The listing builds one solid part. Answer for the finished solid, in the listing's coordinates (mm). Face numbers are marked on the shaded views. A direction names the side the tool comes from. Coordinates: 2 decimals unless noted, no trailing zeros. Order: outer loops, then holes, each group sorted by start corner. A loop starts at its lowest first (then second) coordinate and runs counter-clockwise, first axis right, second up. Notation, with made-up numbers: (-40, 80) -> (10, 80) arc R19 ccw to (10, 105) -> close; hole circle Ø3 at (37.5, 49.5). An arc over 180 degrees is marked (long way). Answer in a Markdown table with one row per item.
```python
from build123d import *

# Parameters (mm, degrees)
F1_DEPTH = 32
F2_R     = 43.740238
F2_R_2   = 35
F3_DEPTH = 88.001
F4_SIZE2 = 10
F4_SIZE  = 10


with BuildPart() as f1:
    # F0 (on Front) → F1 (new body)
    with BuildSketch(Plane.XZ):
        Polygon((-12.5, 32), (-31.5, 32), (-31.5, -19), (-56.5, -19), (-56.5, -32), (-17.5, -32), (-17.5, -15), (17.5, -15), (17.5, -32), (56.5, -32), (56.5, -19), (31.5, -19), (31.5, 32), (12.5, 32), (12.5, -2), (-12.5, -2), align=None)
    extrude(amount=F1_DEPTH)

    # F2 (on face) → F3 (cut, through all)
    with BuildSketch(Plane.YZ.offset(31.5)):
        with Locations((-16, -3)):
            Circle(F2_R)
        with Locations((-16, -3)):
            Circle(F2_R_2, mode=Mode.SUBTRACT)
    extrude(amount=-F3_DEPTH, mode=Mode.SUBTRACT)

    # F4
    f4_edges = [f1.edges().sort_by_distance(p)[0] for p in [
        (-56.5, -32, -25.5),
        (56.5, -32, -25.5),
    ]]
    chamfer(f4_edges, length=F4_SIZE, length2=F4_SIZE2)


solid = f1.part
```
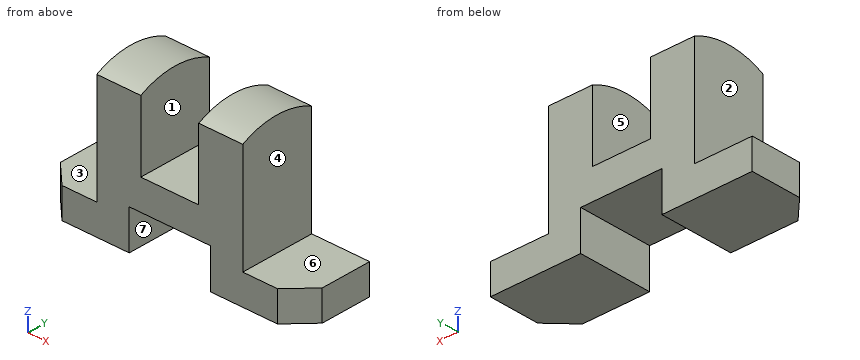
(1) Find the intervals of material crossed by line 1 along X through (y, z) = (-14.5, -18.5); line 2 along X through (y, z) = (-7, 20); line 3 along Z through (x, y) = (34, -25), in increasing order. Write a range as from..to.
Check values:
| item | result |
|---|---|
| line 1 | -31.5..-17.5, 17.5..31.5 |
| line 2 | -31.5..-12.5, 12.5..31.5 |
| line 3 | -32..-19 |
(2) A cutting plane is placed at C-C, the plane z = 15. Determine the outline of the cut face in (x, y), then the cut area to 3 significant figures.
Check values:
| item | result |
|---|---|
| outline | (-31.5, -32) -> (-12.5, -32) -> (-12.5, 0) -> (-31.5, 0) -> close; (12.5, -32) -> (31.5, -32) -> (31.5, 0) -> (12.5, 0) -> close |
| area | 1,220 mm² |
(3) Which of the six approach directions +Z, -Z, +X, -X, +Y, -Y give full straight-line access (tool end or side, diameter ignored) to the marked faces 5, 6 and 7?
Check values:
| item | result |
|---|---|
| face 5 | +Z, +Y, -Y |
| face 6 | +Z, +X, +Y, -Y |
| face 7 | -Z, +Y, -Y |
(4) A cutting plane is placed at A-A, the plane z = -28. Determine the outline of the cut face in (x, y).
Check values:
| item | result |
|---|---|
| outline | (-56.5, -22) -> (-46.5, -32) -> (-17.5, -32) -> (-17.5, 0) -> (-56.5, 0) -> close; (17.5, -32) -> (46.5, -32) -> (56.5, -22) -> (56.5, 0) -> (17.5, 0) -> close |
(5) A cutting plane is placed at D-D, the plane x = -42. Determine the outline of the cut face in (y, z).
Check values:
| item | result |
|---|---|
| outline | (-32, -32) -> (0, -32) -> (0, -19) -> (-32, -19) -> close |
(6) Flat-ended cylindrical pins translate along their axes: pin 1 (16 mm diameter, centred on x = -2, y = -18, fed in from -Z); pin 2 (5 mm diameter, centred on y = -17.5, z = 23, fed in from -X); pin 3 (12.5 mm diameter, centred on x = -3.5, y = -12.5, fed in from +Z). Find the tip coordinate at first contact, or state that the pin passes through.
Check values:
| item | result |
|---|---|
| pin 1 | z = -15 |
| pin 2 | x = -31.5 |
| pin 3 | z = -2 |
(7) For a pull along X with two mould halves and no side action, classify the marked faces 1, 2, 3 and 4 as released by +X, released by -X, zero draft, split by the parting line, or undercut.
Check values:
| item | result |
|---|---|
| face 1 | undercut |
| face 2 | released by -X |
| face 3 | zero draft |
| face 4 | released by +X |
(8) A cutting plane is placed at B-B, the plane y = -10.5. Determine the outline of the cut face in (x, z), then the cut area to 3 significant figures.
Check values:
| item | result |
|---|---|
| outline | (-56.5, -32) -> (-17.5, -32) -> (-17.5, -15) -> (17.5, -15) -> (17.5, -32) -> (56.5, -32) -> (56.5, -19) -> (31.5, -19) -> (31.5, 31.57) -> (12.5, 31.57) -> (12.5, -2) -> (-12.5, -2) -> (-12.5, 31.57) -> (-31.5, 31.57) -> (-31.5, -19) -> (-56.5, -19) -> close |
| area | 3,220 mm² |
